```python
from build123d import *

# Parameters (mm, degrees)
SKETCH1_W                       = 20.480821918
SKETCH1_H                       = 31.9
SKETCH1_R                       = 2.45
BOSS_EXTRUDE1_DEPTH             = 7.5
SKETCH2_W                       = 18.980821918
SKETCH2_H                       = 9.35
CUT_EXTRUDE1_DEPTH              = 6.2
CUT_EXTRUDE2_REACH              = 22.384
SKETCH5_W                       = 5.480821918
SKETCH5_H                       = 31.9
SKETCH3_R                       = 3
SKETCH3_R_2                     = 1.55
BOSS_EXTRUDE4_DEPTH             = 6.2
SKETCH6_W                       = 1.5
SKETCH6_H                       = 15.5
CUT_EXTRUDE3_DEPTH              = 6.2
SKETCH7_W                       = 1.5
SKETCH7_H                       = 18.7
BOSS_EXTRUDE5_DEPTH             = 6.2
FILLET1_R                       = 3
SKETCH8_W                       = 6
SKETCH8_H                       = 4
CUT_EXTRUDE4_DEPTH              = 7.5
FILLET2_R                       = 3
BOSS_EXTRUDE6_REACH             = 21.943
BOSS_EXTRUDE6_DIRECTION_2_REACH = 21.943
SKETCH10_R                      = 3.25
CUT_EXTRUDE6_DEPTH              = 4.5
FILLET3_R                       = 1.5


with BuildPart() as part:
    # Sketch1 → Boss-Extrude1 (new body)
    with BuildSketch(Plane.XY):
        Rectangle(SKETCH1_W, SKETCH1_H)
        with Locations((6.290410959, 12)):
            Circle(SKETCH1_R, mode=Mode.SUBTRACT)
        with Locations((6.290410959, -12)):
            Circle(SKETCH1_R, mode=Mode.SUBTRACT)
    extrude(amount=BOSS_EXTRUDE1_DEPTH)

    # Sketch2 → Cut-Extrude1 (cut)
    with BuildSketch(Plane.XY.offset(7.5)):
        with Locations((-0.75, 4.675)):
            Rectangle(SKETCH2_W, SKETCH2_H)
        with Locations((-0.75, -4.675)):
            Rectangle(SKETCH2_W, SKETCH2_H)
    extrude(amount=-CUT_EXTRUDE1_DEPTH, mode=Mode.SUBTRACT)

    # Cut-Extrude2: up to this face of the body (flat: up to its plane)
    cut_extrude2_end = Plane(part.part.faces().sort_by_distance((-0.385368256, 0, 0))[0])
    # Sketch5 → Cut-Extrude2 (cut, up to the picked face)
    with BuildSketch(Plane.XY.offset(7.5), mode=Mode.PRIVATE) as cut_extrude2_sk1:
        with Locations((-7.5, 0)):
            Rectangle(SKETCH5_W, SKETCH5_H)
    cut_extrude2_tool1 = split(extrude(cut_extrude2_sk1.sketch, amount=-CUT_EXTRUDE2_REACH, mode=Mode.PRIVATE), bisect_by=cut_extrude2_end, keep=Keep.BOTH, mode=Mode.PRIVATE)
    add(cut_extrude2_tool1.solids().sort_by(Axis((-7.5, 0, 7.5), (0, 0, -1)))[0], mode=Mode.SUBTRACT)

    # Sketch3 → Boss-Extrude4 (add)
    # profile 1 of 2: a face of its own
    with BuildSketch(Plane.XY.offset(1.3)):
        with Locations(Location((-1.259589041, 5, 0), (0, 0, 180))):
            Circle(SKETCH3_R)
        with Locations(Location((-1.259589041, 5, 0), (0, 0, 180))):
            Circle(SKETCH3_R_2, mode=Mode.SUBTRACT)
    # profile 2 of 2: a face of its own
    with BuildSketch(Plane.XY.offset(1.3)):
        with Locations(Location((-1.259589041, -5, 0), (0, 0, 180))):
            Circle(SKETCH3_R)
        with Locations(Location((-1.259589041, -5, 0), (0, 0, 180))):
            Circle(SKETCH3_R_2, mode=Mode.SUBTRACT)
    extrude(amount=BOSS_EXTRUDE4_DEPTH)

    # Sketch6 → Cut-Extrude3 (cut)
    with BuildSketch(Plane.XY.offset(7.5)):
        with Locations((9.490410959, 0)):
            Rectangle(SKETCH6_W, SKETCH6_H)
    extrude(amount=-CUT_EXTRUDE3_DEPTH, mode=Mode.SUBTRACT)

    # Sketch7 → Boss-Extrude5 (add)
    with BuildSketch(Plane.XY.offset(1.3)):
        with Locations((-4.009589041, 0)):
            Rectangle(SKETCH7_W, SKETCH7_H)
    extrude(amount=BOSS_EXTRUDE5_DEPTH)

    # Fillet1
    fillet1_edges = [part.edges().sort_by_distance(p)[0] for p in [
        (10.240410959, 15.95, 3.75),
        (10.240410959, -15.95, 3.75),
    ]]
    fillet(fillet1_edges, radius=FILLET1_R)

    # Sketch8 → Cut-Extrude4 (cut)
    with BuildSketch(Plane.XY.offset(7.5)):
        with Locations((-1.759589041, 13.95)):
            Rectangle(SKETCH8_W, SKETCH8_H)
        with Locations((-1.759589041, -13.95)):
            Rectangle(SKETCH8_W, SKETCH8_H)
    extrude(amount=-CUT_EXTRUDE4_DEPTH, mode=Mode.SUBTRACT)

    # Fillet2
    fillet2_edges = [part.edges().sort_by_distance(p)[0] for p in [
        (1.240410959, 15.95, 3.75),
        (-4.759589041, 11.95, 3.75),
        (1.240410959, -15.95, 3.75),
        (-4.759589041, -11.95, 3.75),
    ]]
    fillet(fillet2_edges, radius=FILLET2_R)

    # Boss-Extrude6: up to this face of the body (flat: up to its plane)
    boss_extrude6_end = Plane(part.part.faces().sort_by_distance((5.740410959, -15.597493262, 7.5))[0])
    # Sketch11 → Boss-Extrude6 (add, up to the picked face)
    with BuildSketch(Plane.XY.offset(1.3), mode=Mode.PRIVATE) as boss_extrude6_sk1:
        with BuildLine():
            Line((-3.259589041, 7.236067977), (-3.259589041, 7.75))
            Line((-3.259589041, 7.75), (-3.259589041, 9.35))
            Line((-3.259589041, 9.35), (8.740410959, 9.35))
            Line((8.740410959, 9.35), (8.740410959, 7.75))
            Line((8.740410959, 7.75), (-0.06063116, 7.75))
            ThreePointArc((-0.06063116, 7.75), (-1.735455251, 7.962018121), (-3.259589041, 7.236067977))
        make_face()
    boss_extrude6_tool1 = split(extrude(boss_extrude6_sk1.sketch, amount=BOSS_EXTRUDE6_REACH, mode=Mode.PRIVATE), bisect_by=boss_extrude6_end, keep=Keep.BOTH, mode=Mode.PRIVATE)
    # Sketch11 → Boss-Extrude6 (add, up to the picked face)
    with BuildSketch(Plane.XY.offset(1.3), mode=Mode.PRIVATE) as boss_extrude6_sk2:
        with BuildLine():
            Line((-3.259589041, -7.75), (-3.259589041, -9.35))
            Line((-3.259589041, -9.35), (8.740410959, -9.35))
            Line((8.740410959, -9.35), (8.740410959, -7.75))
            Line((8.740410959, -7.75), (-0.06063116, -7.75))
            ThreePointArc((-0.06063116, -7.75), (-1.735455251, -7.962018121), (-3.259589041, -7.236067977))
            Line((-3.259589041, -7.236067977), (-3.259589041, -7.75))
        make_face()
    boss_extrude6_tool2 = split(extrude(boss_extrude6_sk2.sketch, amount=BOSS_EXTRUDE6_REACH, mode=Mode.PRIVATE), bisect_by=boss_extrude6_end, keep=Keep.BOTH, mode=Mode.PRIVATE)
    add(boss_extrude6_tool1.solids().sort_by(Axis((2.770321, 8.555653, 1.3), (0, 0, 1)))[0])
    add(boss_extrude6_tool2.solids().sort_by(Axis((2.770321, -8.555653, 1.3), (0, 0, 1)))[0])

    # Boss-Extrude6 direction 2: up to this face of the body (flat: up to its plane)
    boss_extrude6_direction_2_end = Plane(part.part.faces().sort_by_distance((2.964227546, 0, 0))[0])
    # Sketch11 → Boss-Extrude6 direction 2 (add, up to the picked face)
    with BuildSketch(Plane.XY.offset(1.3), mode=Mode.PRIVATE) as boss_extrude6_direction_2_sk1:
        with BuildLine():
            Line((-3.259589041, 7.236067977), (-3.259589041, 7.75))
            Line((-3.259589041, 7.75), (-3.259589041, 9.35))
            Line((-3.259589041, 9.35), (8.740410959, 9.35))
            Line((8.740410959, 9.35), (8.740410959, 7.75))
            Line((8.740410959, 7.75), (-0.06063116, 7.75))
            ThreePointArc((-0.06063116, 7.75), (-1.735455251, 7.962018121), (-3.259589041, 7.236067977))
        make_face()
    boss_extrude6_direction_2_tool1 = split(extrude(boss_extrude6_direction_2_sk1.sketch, amount=-BOSS_EXTRUDE6_DIRECTION_2_REACH, mode=Mode.PRIVATE), bisect_by=boss_extrude6_direction_2_end, keep=Keep.BOTH, mode=Mode.PRIVATE)
    # Sketch11 → Boss-Extrude6 direction 2 (add, up to the picked face)
    with BuildSketch(Plane.XY.offset(1.3), mode=Mode.PRIVATE) as boss_extrude6_direction_2_sk2:
        with BuildLine():
            Line((-3.259589041, -7.75), (-3.259589041, -9.35))
            Line((-3.259589041, -9.35), (8.740410959, -9.35))
            Line((8.740410959, -9.35), (8.740410959, -7.75))
            Line((8.740410959, -7.75), (-0.06063116, -7.75))
            ThreePointArc((-0.06063116, -7.75), (-1.735455251, -7.962018121), (-3.259589041, -7.236067977))
            Line((-3.259589041, -7.236067977), (-3.259589041, -7.75))
        make_face()
    boss_extrude6_direction_2_tool2 = split(extrude(boss_extrude6_direction_2_sk2.sketch, amount=-BOSS_EXTRUDE6_DIRECTION_2_REACH, mode=Mode.PRIVATE), bisect_by=boss_extrude6_direction_2_end, keep=Keep.BOTH, mode=Mode.PRIVATE)
    add(boss_extrude6_direction_2_tool1.solids().sort_by(Axis((2.770321, 8.555653, 1.3), (0, 0, -1)))[0])
    add(boss_extrude6_direction_2_tool2.solids().sort_by(Axis((2.770321, -8.555653, 1.3), (0, 0, -1)))[0])

    # Sketch10 → Cut-Extrude6 (cut)
    with BuildSketch(Plane(origin=(0, 0, 0), x_dir=(-1, 0, 0), z_dir=(0, 0, -1))):
        with Locations((-6.290410959, 12)):
            Circle(SKETCH10_R)
        with Locations((-6.290410959, -12)):
            Circle(SKETCH10_R)
    extrude(amount=-CUT_EXTRUDE6_DEPTH, mode=Mode.SUBTRACT)

    # Fillet3
    fillet3_edges = [part.edges().sort_by_distance(p)[0] for p in [
        (1.265413056, 3.380010984, 1.3),
        (1.265413056, -3.380010984, 1.3),
    ]]
    fillet(fillet3_edges, radius=FILLET3_R)


solid = part.part
```
The listing builds one solid part. Answer for the finished solid, in the listing's coordinates (mm). A direction names the side the tool comes from. Round coordinates to 2 decimals unless told otherwise and drop trailing zeros. Write each loop counter-clockwise with the first axis right and the second up, starting at its lowest first coordinate (ties: lowest second). Pieces come first, ordered by that corner, then holes. Notation, with made-up numbers: (-11, -1) -> (30, -1) arc R30 ccw to (30, 26) -> close; hole circle Ø4 at (36.25, -27). An arc over 180 degrees is marked (long way). Answer as a JSON object with one key per item and string values. Group by question number.
Q1. Straight lines are drawn through the part: line 1 along Y through (x, z) = (6.25, 2.5); line 2 along X through (y, z) = (-5, 5.75); line 3 along Y through (x, z) = (4.75, 6.75). For each, find the intervals that lie inside material, in ascending order.
Q2. Section A-A (z = 5.5) is taken. Write down the section's boundary in (x, y).
Q3. Which of the six approach directions +Z, -Z, +X, -X, +Y, -Y give full straight-line access (tool end or side, diameter ignored) to faces 5 (the face through (3.2, 13, 2.2)), 6 (the face through (-1.975, 6.375, 4.357)), 7 (the face through (1.24, -12.5, 3.8)), 8 (the face through (0, 11.95, 4))?
Q4. Section C-C (z = 1) is taken. Write down the section's boundary in (x, y), plus the area to 3 significant figures.
Q5. Section D-D (y = -5) is taken. Write down the section's boundary in (x, z), plus the area to 3 significant figures.
Q6. Each of these flat-tipped pins is pushed along its axis until it touches: pin 1 Ø8 at (x, y) = (6.29, -12) entering from +Z; pin 2 Ø3 at (x, y) = (6.29, 12) entering from -Z; pin 3 Ø1 at (x, z) = (-3, 5) entering from -Y; pin 4 Ø1.5 at (x, y) = (7, 1.5) entering from +Z. Where does it stop, or does it pass through?
Q7. Determine the mould class of faces 1 (the face through (7.421, 9.826, 5.979)), 2 (the face through (0, -11.95, 4)), 3 (the face through (-1.975, -3.625, 4.357)), 4 (the face through (9.385, 15.048, 3.802)) for opening direction Y: pulls with the +Y half, pulls with the -Y half, needs draft (parallel to the pull), parting line crosses it, or undercut.
Q8. Section B-B (y = 11) is taken. Write down the section's boundary in (x, z).
Check values:
{
 "1": {"line 1": "-15.95 to -15.25, -8.75 to -7.75, 7.75 to 8.75, 15.25 to 15.95", "line 2": "-4.76 to -2.81, 0.29 to 1.74", "line 3": "-15.95 to -13.91, -10.09 to -7.75, 7.75 to 10.09, 13.91 to 15.95"},
 "2": {"outline": "(-4.76, -8.95) arc R3 ccw to (-1.76, -11.95) -> (1.24, -11.95) -> (1.24, -12.95) arc R3 ccw to (4.24, -15.95) -> (7.24, -15.95) arc R3 ccw to (10.24, -12.95) -> (10.24, -7.75) -> (-0.06, -7.75) arc R3 ccw (long way) to (-3.26, -2.76) -> (-3.26, 2.76) arc R3 ccw (long way) to (-0.06, 7.75) -> (10.24, 7.75) -> (10.24, 12.95) arc R3 ccw to (7.24, 15.95) -> (4.24, 15.95) arc R3 ccw to (1.24, 12.95) -> (1.24, 11.95) -> (-1.76, 11.95) arc R3 ccw to (-4.76, 8.95) -> close; hole circle Ø3.1 at (-1.26, -5); hole circle Ø3.1 at (-1.26, 5); hole circle Ø4.9 at (6.29, -12); hole circle Ø4.9 at (6.29, 12)"},
 "3": {"face 5": "-Z", "face 6": "+Z", "face 7": "+Z, -Z, -X, -Y", "face 8": "+Z, -Z, -X, +Y"},
 "4": {"outline": "(-4.76, -8.95) arc R3 ccw to (-1.76, -11.95) -> (1.24, -11.95) -> (1.24, -12.95) arc R3 ccw to (4.24, -15.95) -> (7.24, -15.95) arc R3 ccw to (10.24, -12.95) -> (10.24, 12.95) arc R3 ccw to (7.24, 15.95) -> (4.24, 15.95) arc R3 ccw to (1.24, 12.95) -> (1.24, 11.95) -> (-1.76, 11.95) arc R3 ccw to (-4.76, 8.95) -> close; hole circle Ø6.5 at (6.29, -12); hole circle Ø6.5 at (6.29, 12)", "area": "353 mm^2"},
 "5": {"outline": "(-4.76, 0) -> (10.24, 0) -> (10.24, 1.3) -> (3.24, 1.3) arc R1.5 cw to (1.74, 2.8) -> (1.74, 7.5) -> (0.29, 7.5) -> (0.29, 1.3) -> (-2.81, 1.3) -> (-2.81, 7.5) -> (-4.76, 7.5) -> close", "area": "41.1 mm^2"},
 "6": {"pin 1": "z = 7.5", "pin 2": "through", "pin 3": "y = -11.86", "pin 4": "z = 1.3"},
 "7": {"face 1": "undercut", "face 2": "pulls with the -Y half", "face 3": "undercut", "face 4": "pulls with the +Y half"},
 "8": {"outline": "(-3.95, 0) -> (3.2, 0) -> (3.2, 4.5) -> (4.05, 4.5) -> (4.05, 7.5) -> (-3.95, 7.5) -> close; (8.53, 4.5) -> (9.38, 4.5) -> (9.38, 0) -> (10.24, 0) -> (10.24, 7.5) -> (8.53, 7.5) -> close"}
}
